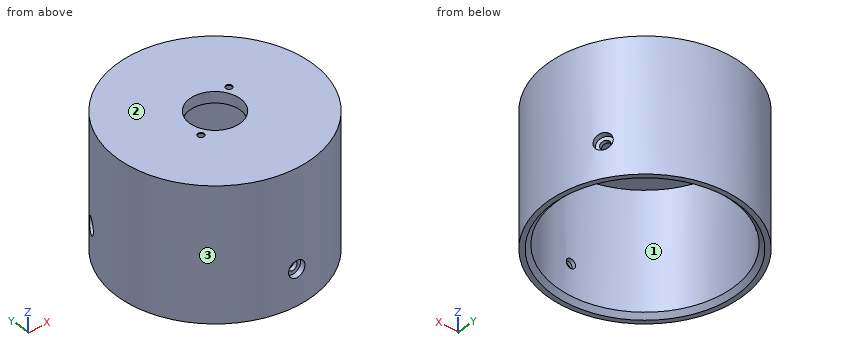
```python
from build123d import *

# Parameters (mm, degrees)
SKETCH1_R                                   = 28.0035
SKETCH1_R_2                                 = 25.3365
BOSS_EXTRUDE1_DEPTH                         = 38.1
BOSS_EXTRUDE2_START                         = -3.175
SKETCH10_R                                  = 28.0035
BOSS_EXTRUDE2_DEPTH                         = 3.175
CBORE_START                                 = -28.003500075
CBORE_FOR_2_PAN_HEAD_MACHINE_SCREW1_OUT_R   = 2.38125
CBORE_FOR_2_PAN_HEAD_MACHINE_SCREW1_DEPTH   = 1.574800075
CBORE_START_2                               = -26.4287
CBORE_FOR_2_PAN_HEAD_MACHINE_SCREW1_2_O_R   = 1.35255
CBORE_FOR_2_PAN_HEAD_MACHINE_SCREW1_2_DEPTH = 1.128327756
CBORE_START_3                               = 26.4287
CBORE_FOR_2_PAN_HEAD_MACHINE_SCREW2_OUT_R   = 2.38125
CBORE_FOR_2_PAN_HEAD_MACHINE_SCREW2_DEPTH   = 1.574800075
CBORE_START_4                               = 25.300372244
CBORE_FOR_2_PAN_HEAD_MACHINE_SCREW2_2_O_R   = 1.35255
CBORE_FOR_2_PAN_HEAD_MACHINE_SCREW2_2_DEPTH = 1.128327756
CBORE_START_5                               = -28.003500101
CBORE_FOR_2_PAN_HEAD_MACHINE_SCREW3_OUT_R   = 2.38125
CBORE_FOR_2_PAN_HEAD_MACHINE_SCREW3_DEPTH   = 1.574800101
CBORE_FOR_2_PAN_HEAD_MACHINE_SCREW3_2_O_R   = 1.35255
CBORE_FOR_2_PAN_HEAD_MACHINE_SCREW3_2_DEPTH = 1.128327733
CUT_EXTRUDE1_REACH                          = 56.955
SKETCH20_R                                  = 7.27
HOLE1_AT_2_COUNT                            = 2
HOLE1_AT_2_PITCH                            = 19
F_0_CLEARANCE_HOLE1_D                       = 1.8542
CHAMFER1_SIZE                               = 1.27


# Read off the part's stored shape, not the designer's step: CBORE for #2 Pan Head Machine Screw1, CBORE for #2 Pan Head Machine Screw2, CBORE for #2 Pan Head Machine Screw3
with BuildPart() as part:
    # Sketch1 → Boss-Extrude1 (new body)
    with BuildSketch(Plane.XY):
        with Locations(Location((0, 0, 0), (0, 0, 180))):
            Circle(SKETCH1_R)
        with Locations(Location((0, 0, 0), (0, 0, 180))):
            Circle(SKETCH1_R_2, mode=Mode.SUBTRACT)
    extrude(amount=BOSS_EXTRUDE1_DEPTH)

    # Sketch10 → Boss-Extrude2 (add)
    with BuildSketch(Plane.XY.offset(38.1).offset(BOSS_EXTRUDE2_START)):
        with Locations(Location((0, 0, 0), (0, 0, 180))):
            Circle(SKETCH10_R)
    extrude(amount=BOSS_EXTRUDE2_DEPTH)

    # CBORE for #2 Pan Head Machine Screw1 out → CBORE for #2 Pan Head Machine Screw1 (cut)
    with BuildSketch(Plane(origin=(0, 0, 0), x_dir=(0.500000000000004, 0.8660254037844363, 0), z_dir=(0.8660254037844363, -0.5000000000000042, 0)).offset(CBORE_START)):
        with Locations((0, 10.2108)):
            Circle(CBORE_FOR_2_PAN_HEAD_MACHINE_SCREW1_OUT_R)
    extrude(amount=CBORE_FOR_2_PAN_HEAD_MACHINE_SCREW1_DEPTH, mode=Mode.SUBTRACT)

    # CBORE for _2 Pan Head Machine Screw1 2 o → CBORE for _2 Pan Head Machine Screw1 2 (cut)
    with BuildSketch(Plane(origin=(0, 0, 0), x_dir=(0.500000000000004, 0.8660254037844363, 0), z_dir=(0.8660254037844363, -0.5000000000000042, 0)).offset(CBORE_START_2)):
        with Locations((0, 10.2108)):
            Circle(CBORE_FOR_2_PAN_HEAD_MACHINE_SCREW1_2_O_R)
    extrude(amount=CBORE_FOR_2_PAN_HEAD_MACHINE_SCREW1_2_DEPTH, mode=Mode.SUBTRACT)

    # CBORE for #2 Pan Head Machine Screw2 out → CBORE for #2 Pan Head Machine Screw2 (cut)
    with BuildSketch(Plane(origin=(0, 0, 0), x_dir=(0.500000000000004, -0.8660254037844363, 0), z_dir=(0.8660254037844363, 0.5000000000000042, 0)).offset(CBORE_START_3)):
        with Locations((0, -10.2108)):
            Circle(CBORE_FOR_2_PAN_HEAD_MACHINE_SCREW2_OUT_R)
    extrude(amount=CBORE_FOR_2_PAN_HEAD_MACHINE_SCREW2_DEPTH, mode=Mode.SUBTRACT)

    # CBORE for _2 Pan Head Machine Screw2 2 o → CBORE for _2 Pan Head Machine Screw2 2 (cut)
    with BuildSketch(Plane(origin=(0, 0, 0), x_dir=(0.500000000000004, -0.8660254037844363, 0), z_dir=(0.8660254037844363, 0.5000000000000042, 0)).offset(CBORE_START_4)):
        with Locations((0, -10.2108)):
            Circle(CBORE_FOR_2_PAN_HEAD_MACHINE_SCREW2_2_O_R)
    extrude(amount=CBORE_FOR_2_PAN_HEAD_MACHINE_SCREW2_2_DEPTH, mode=Mode.SUBTRACT)

    # CBORE for #2 Pan Head Machine Screw3 out → CBORE for #2 Pan Head Machine Screw3 (cut)
    with BuildSketch(Plane(origin=(0, 0, 0), x_dir=(1, 0, 0), z_dir=(0, 1, 0)).offset(CBORE_START_5)):
        with Locations((0, -10.2108)):
            Circle(CBORE_FOR_2_PAN_HEAD_MACHINE_SCREW3_OUT_R)
    extrude(amount=CBORE_FOR_2_PAN_HEAD_MACHINE_SCREW3_DEPTH, mode=Mode.SUBTRACT)

    # CBORE for _2 Pan Head Machine Screw3 2 o → CBORE for _2 Pan Head Machine Screw3 2 (cut)
    with BuildSketch(Plane(origin=(0, 0, 0), x_dir=(1, 0, 0), z_dir=(0, 1, 0)).offset(CBORE_START_2)):
        with Locations((0, -10.2108)):
            Circle(CBORE_FOR_2_PAN_HEAD_MACHINE_SCREW3_2_O_R)
    extrude(amount=CBORE_FOR_2_PAN_HEAD_MACHINE_SCREW3_2_DEPTH, mode=Mode.SUBTRACT)

    # Sketch20 → Cut-Extrude1 (cut, up to next)
    with BuildSketch(Plane.XY.offset(38.1), mode=Mode.PRIVATE) as cut_extrude1_sk1:
        Circle(SKETCH20_R)
    cut_extrude1_tool1 = extrude(cut_extrude1_sk1.sketch, amount=-CUT_EXTRUDE1_REACH, mode=Mode.PRIVATE) & part.part
    add(cut_extrude1_tool1.solids().sort_by_distance((0, 0, 38.1))[0], mode=Mode.SUBTRACT)

    # Sketch22 → Hole1 (revolve, cut)
    with BuildSketch(Plane(origin=(8.195734173, 4.804158758, 34.925), x_dir=(0, 1, 0), z_dir=(1, 0, 0))):
        Polygon((0, 0), (0, 2.921), (1.4986, 2.921), (1.6383, 0), align=None)
    hole1 = revolve(axis=Axis((8.195734173, 4.804158758, 144.925), (0, 0, -1)), mode=Mode.SUBTRACT)

    # Hole1 at 2: Hole1 ×2
    with Locations(*[Vector(-0.8627088602819588, -0.5057009218807137, 0) * (i * HOLE1_AT_2_PITCH) for i in range(1, HOLE1_AT_2_COUNT)]):
        add(hole1, mode=Mode.SUBTRACT)

    # #0 Clearance Hole1 (through all)
    with Locations(Plane(origin=(0, 0, 34.925), x_dir=(-1, 0, 0), z_dir=(0, 0, -1))):
        with Locations((-8.195734173, 4.804158758), (8.195734173, -4.804158758)):
            Hole(F_0_CLEARANCE_HOLE1_D / 2)

    # Chamfer1
    chamfer1_edges = [part.edges().sort_by_distance(p)[0] for p in [
        (25.3365, 0, 0),
    ]]
    chamfer(chamfer1_edges, length=CHAMFER1_SIZE)


solid = part.part
```
Work out the finished part from the listing and answer in its coordinate system (mm). Face numbers are marked on the shaded views. Coordinates: 2 decimals unless noted, no trailing zeros. Loops run counter-clockwise (first coordinate to the right, second up) from the corner with the lowest first, then second, coordinate; pieces in that order, holes last.
1) For a pull along X with two mould halves and no side action, classify the marked faces 1, 2 and 3 as +X half, -X half, draft (parallel to the pull), parting line (faces both ways), or undercut.
Results:
face 1: undercut
face 2: draft
face 3: parting line
2) Consider probe 1 along Y at (x, z) = (0.5, 23.5); probe 2 along Z at (x, y) = (11, 20) (3 decimals); probe 3 along Y at (x, z) = (6, 26). Determine where each line is inside the solid, lowest interval first.
Results:
probe 1: y = -28 to -25.33, 25.33 to 28
probe 2: z = 34.925 to 38.1
probe 3: y = -27.35 to -24.62, 24.62 to 27.35
3) Section B-B (x = 0) is taken. Give the vertices of the cut face in (y, z) (1 decimal).
Results:
outline: (-28, 0) - (-26.6, 0) - (-25.3, 1.3) - (-25.3, 8.9) - (-26.4, 8.9) - (-26.4, 7.8) - (-28, 7.8) - close; (-28, 12.6) - (-26.4, 12.6) - (-26.4, 11.6) - (-25.3, 11.6) - (-25.3, 34.9) - (-7.3, 34.9) - (-7.3, 38.1) - (-28, 38.1) - close; (7.3, 34.9) - (25.3, 34.9) - (25.3, 1.3) - (26.6, 0) - (28, 0) - (28, 38.1) - (7.3, 38.1) - close
4) Flat-ended cylindrical pins translate along their axes: pin 1 (12 mm diameter, centred on x = -0.5, y = -16.5, fed in from -Z) (3 decimals); pin 2 (4 mm diameter, centred on y = -3.5, z = 23.5, fed in from +X); pin 3 (6 mm diameter, centred on y = -15, z = 12.5, fed in from +X). Find the tip coordinate at first contact, or state that the pin passes through.
Results:
pin 1: stops at z = 34.925
pin 2: stops at x = 27.96
pin 3: stops at x = 25.3
5) Section A-A (y = 0) is taken. Give the vertices of the cut face in (x, z) (1 decimal), plus the area to 3 significant figures.
Results:
outline: (-28, 0) - (-26.6, 0) - (-25.3, 1.3) - (-25.3, 34.9) - (-7.3, 34.9) - (-7.3, 38.1) - (-28, 38.1) - close; (7.3, 34.9) - (25.3, 34.9) - (25.3, 1.3) - (26.6, 0) - (28, 0) - (28, 38.1) - (7.3, 38.1) - close
area: 316 mm2
6) Section C-C (z = 18) is taken. Give the vertices of the cut face in (x, y), plus the area to 3 significant figures.
Results:
outline: circle Ø56.01 at (0, 0); hole circle Ø50.67 at (0, 0)
area: 447 mm2
